```python
from build123d import *

# Parameters (mm, degrees)
SKETCH_1_W                  = 70
SKETCH_1_H                  = 220
EXTRUDE_1_DEPTH             = 40
HOLE_WIZARD_M81_D           = 9
HOLE_WIZARD_M81_CBORE_D     = 15
HOLE_WIZARD_M81_CBORE_DEPTH = 8.6
EXTRUDE_2_DEPTH             = 10
HOLE_WIZARD_M61_D           = 5


with BuildPart() as part:
    # Эскиз1 → Бобышка-Вытянуть1 (new body)
    with BuildSketch(Plane(origin=(0, 0, 0), x_dir=(1, 0, 0), z_dir=(0, 1, 0))):
        Rectangle(SKETCH_1_W, SKETCH_1_H)
    extrude(amount=EXTRUDE_1_DEPTH)

    # Цековка для  винта с внутренним шестигранником M81 (through all)
    with Locations(Plane(origin=(0, 40, 0), x_dir=(1, 0, 0), z_dir=(0, 1, 0))):
        with Locations((-28.5, -46), (28.5, -46), (28.5, -91), (-28.5, -91)):
            hole_wizard_m81 = CounterBoreHole(HOLE_WIZARD_M81_D / 2, HOLE_WIZARD_M81_CBORE_D / 2, HOLE_WIZARD_M81_CBORE_DEPTH)

    # Зеркальное отражение1: Цековка для  винта с внутренним шестигранником M81 across plane
    add(hole_wizard_m81.mirror(Plane.XY), mode=Mode.SUBTRACT)

    # Эскиз4 → Бобышка-Вытянуть2 (add, symmetric)
    with BuildSketch(Plane(origin=(0, 0, 0), x_dir=(0, 0, -1), z_dir=(1, 0, 0))):
        Polygon((100, 40), (100, 400), (45, 400), (45, 360), (53, 360), (53, 390), (64, 390), (64, 270), (53, 270), (53, 300), (45, 300), (-100, 40), align=None)
    extrude(amount=EXTRUDE_2_DEPTH, both=True)

    # Отверстие обработанное метчиком M61 (through all)
    with Locations(Plane(origin=(35, 0, 0), x_dir=(0, 0, -1), z_dir=(1, 0, 0))):
        with Locations((-30, 20), (30, 20)):
            Hole(HOLE_WIZARD_M61_D / 2)


solid = part.part
```
Check sheet for the modelled part. Datum: model origin and axes. Units: mm. A direction names the side the tool comes from. Round coordinates to 2 decimals unless told otherwise and drop trailing zeros. Order: outer loops, then holes, each group sorted by start corner. A loop starts at its lowest first (then second) coordinate and runs counter-clockwise, first axis right, second up. Notation, with made-up numbers: (53.5, 5.5) -> (74.5, 5.5) arc R29 cw to (74.5, 28.5) -> close; hole circle Ø11 at (39.25, -3.5). An arc over 180 degrees is marked (long way). Use CSV: the item, a comma, the result in double quotes.
(1) Cross-section at B-B (y = 366). Record the boundary of the cut face in (x, z), and give its area (3 significant figures).
Worked out:
outline,"(-10, -100) -> (10, -100) -> (10, -64) -> (-10, -64) -> close; (-10, -53) -> (10, -53) -> (10, -45) -> (-10, -45) -> close"
area,"880 mm²"
(2) Cross-section at C-C (x = -14). Record the boundary of the cut face in (y, z), and give its area (3 significant figures).
Worked out:
outline,"(0, -110) -> (40, -110) -> (40, 110) -> (0, 110) -> close; hole circle Ø5 at (20, -30); hole circle Ø5 at (20, 30)"
area,"8,760 mm²"
(3) Draft check along X on faces 5 (the face through (0, 285, -53)), 6 (the face through (29.09, 15.48, -86.54)), 7 (the face through (-35, 20, 2)). Enter one of: pulls with the +X half, pulls with the -X half, needs draft (parallel to the pull), parting line crosses it, or undercut.
Worked out:
face 5,"needs draft"
face 6,"undercut"
face 7,"pulls with the -X half"
(4) Tool access check on faces 1 (the face through (0, 380, -45)), 2 (the face through (0, 375, -53)), 3 (the face through (-21, 36, -46)), 4 (the face through (0, 360, -49)). Record the directions out of +Z, -Z, +X, -X, +Y, -Y that give a thin tool (end or side, any length) a straight path to the whole face; none if there is none.
Worked out:
face 1,"+Z, +X, -X, +Y"
face 2,"+X, -X"
face 3,"+Y"
face 4,"+Z, +X, -X"
(5) Depth check by flat-ended pin: pin 1 (8 mm diameter, centred on y = 73.5, z = 31, fed in from -X); pin 2 (1 mm diameter, centred on x = -6, z = 45, fed in from +Y); pin 3 (16 mm diameter, centred on x = -4, y = 187.5, fed in from -Z). Enter the tip coordinate at first touch or a pass-through.
Worked out:
pin 1,"x = -10"
pin 2,"y = 139.52"
pin 3,"z = -100"
(6) Cross-section at D-D (z = -18). Record the boundary of the cut face in (x, y), and give its area (3 significant figures).
Worked out:
outline,"(-35, 0) -> (35, 0) -> (35, 40) -> (10, 40) -> (10, 251.59) -> (-10, 251.59) -> (-10, 40) -> (-35, 40) -> close"
area,"7,030 mm²"
(7) Material ranges on line 1 along X through (y, z) = (25, -91); line 2 along Z through (x, y) = (28.5, 36); line 3 along Z through (x, y) = (5.5, 345.5), recorded low to high. Write a range as from..to.
Worked out:
line 1,"-35..-33, -24..24, 33..35"
line 2,"-110..-98.5, -83.5..-53.5, -38.5..38.5, 53.5..83.5, 98.5..110"
line 3,"-100..-64"
(8) Cross-section at A-A (z = -91). Record the boundary of the cut face in (x, y), and give its area (3 significant figures).
Worked out:
outline,"(-35, 0) -> (-33, 0) -> (-33, 31.4) -> (-35, 31.4) -> close; (-24, 0) -> (24, 0) -> (24, 31.4) -> (21, 31.4) -> (21, 40) -> (10, 40) -> (10, 400) -> (-10, 400) -> (-10, 40) -> (-21, 40) -> (-21, 31.4) -> (-24, 31.4) -> close; (33, 0) -> (35, 0) -> (35, 31.4) -> (33, 31.4) -> close"
area,"9,190 mm²"
